from build123d import *

# Parameters (mm, degrees)
P_IDAT_VYSUNUT_M1_DEPTH  = 3
P_IDAT_VYSUNUT_M2_DEPTH  = 2
ZAOBLIT4_R               = 1
SKICA2_W                 = 4
SKICA2_H                 = 2
ODEBRAT_VYSUNUT_M2_DEPTH = 0.8
SKICA3_W                 = 4
SKICA3_H                 = 2
ODEBRAT_VYSUNUT_M3_DEPTH = 0.8


with BuildPart() as part:
    # Skica1 → P_idat vysunut_m1 (new body)
    with BuildSketch(Plane(origin=(0, 0, 0), x_dir=(1, 0, 0), z_dir=(0, 1, 0))):
        Polygon((-118.143750166, 15), (-118.143750166, 0), (-68.779346971, 32.313398106), (-16.32734533, 12.51119421), (-26.593132493, 30.830954414), (-20.343228113, 42.230019956), (0, 37.22), (0, 69.22), (-39.317553332, 46.52), (-78.635106664, 69.22), (-118.143185584, 46.41), (-118.143185584, 33.5570142), (-107.643750166, 37.378496169), (-107.643750166, 24.278496169), (-128.093750166, 24.278496169), (-128.093750166, 11.378496169), align=None)
    extrude(amount=P_IDAT_VYSUNUT_M1_DEPTH)

    # Skica1_5 → P_idat vysunut_m2 (add)
    with BuildSketch(Plane(origin=(0, 0, 0), x_dir=(1, 0, 0), z_dir=(0, 1, 0))):
        Polygon((-68.779346971, 32.313398106), (-118.143750166, 0), (0, 0), (0, 15), (9.950504516, 11.37831254), (9.950504516, 24.27831254), (-10.5, 24.27831254), (-10.5, 37.37831254), (0, 33.55662508), (0, 37.22), (-20.343228113, 42.230019956), (-26.593132493, 30.830954414), (-16.32734533, 12.51119421), align=None)
    extrude(amount=P_IDAT_VYSUNUT_M2_DEPTH)

    # Zaoblit4
    zaoblit4_edges = [part.edges().sort_by_distance(p)[0] for p in [
        (-118.143750166, 1.5, -15),
        (-128.093750166, 1.5, -11.378496169),
        (-128.093750166, 1.5, -24.278496169),
        (-107.643750166, 1.5, -24.278496169),
        (-107.643750166, 1.5, -37.378496169),
        (-118.143185584, 1.5, -33.5570142),
        (-10.5, 1, -24.27831254),
        (-10.5, 1, -37.37831254),
        (0, 1, -33.55662508),
        (0, 1, -15),
        (9.950504516, 1, -11.37831254),
        (9.950504516, 1, -24.27831254),
    ]]
    fillet(zaoblit4_edges, radius=ZAOBLIT4_R)

    # Skica2 → Odebrat vysunut_m2 (cut)
    with BuildSketch(Plane(origin=(0, 3, 0), x_dir=(1, 0, 0), z_dir=(0, 1, 0))):
        with Locations((-105.643750166, 32.914422166)):
            Rectangle(SKICA2_W, SKICA2_H)
        with Locations((-126.093750166, 20.342570172)):
            Rectangle(SKICA2_W, SKICA2_H)
        with Locations((-105.643750166, 28.314422166)):
            Rectangle(SKICA2_W, SKICA2_H)
    extrude(amount=-ODEBRAT_VYSUNUT_M2_DEPTH, mode=Mode.SUBTRACT)

    # Skica3 → Odebrat vysunut_m3 (cut)
    with BuildSketch(Plane(origin=(0, 2, 0), x_dir=(1, 0, 0), z_dir=(0, 1, 0))):
        with Locations((7.950504516, 15.742386544)):
            Rectangle(SKICA3_W, SKICA3_H)
    extrude(amount=-ODEBRAT_VYSUNUT_M3_DEPTH, mode=Mode.SUBTRACT)


solid = part.part
Part model, mm, in its own coordinate system. A direction names the side the tool comes from. Coordinates: 2 decimals unless noted, no trailing zeros. Loops run counter-clockwise (first coordinate to the right, second up) from the corner with the lowest first, then second, coordinate; pieces in that order, holes last. Notation, with made-up numbers: (74.25, -39.5) -> (132.25, -39.5) arc R3 ccw to (132.25, -34.5) -> close; hole circle Ø1 at (-19, 8.5). An arc over 180 degrees is marked (long way). Use a Markdown table: item, result. Add a question column.
Item 1: Which spindle directions (+Z, -Z, +X, -X, +Y, -Y) get a long thin tool onto all of the face, cutting with end or side? Do faces 1 (the flat face through (-5.305, 0.986, -35.487)), 2 (the flat face through (-123.17, 1.48, -13.17)), 3 (the flat face through (-93.81, 2.49, -15.93)). Say none if no direction does.
Item 2: Band-saw the part on C-C on x = -42.5. Write the cut outline in (y, z), plus the area to 3 significant figures.
Item 3: Pull direction X, two halves, no side cores. Call faces 4 (the flat face through (-60, 0, -27)), 5 (the flat face through (-107.644, 1, -31)), 6 (the flat face through (-21.388, 2.493, -21.543)), 7 (the flat face through (-118.143, 1, -41)): +X half, -X half, draft (parallel to the pull), parting line (faces both ways), or undercut.
Item 4: Flat gauge pins, fed straight in: P1, Ø0.9, axis at x = -106.5, y = 2.5, coming from the -Z side; P2, Ø0.6, axis at x = 1.5, y = 1, coming from the -Z side; P3, Ø1.5, axis at y = 1.5, z = -30, coming from the -X side. Where does each tip first touch, or does it go through?
Item 5: Band-saw the part on D-D on z = -5. Write the cut outline in (x, y), plus the area to 3 significant figures.
Item 6: Band-saw the part on B-B on z = -61.5. Write the cut outline in (x, y).
Item 7: Probe probe 1 along Y at (x, z) = (-39, -19); probe 2 along X at (y, z) = (2.45, -43); probe 3 along Z at (x, y) = (-114.5, 0.25). List the from-to ranges inside material, lowest first.
Geometry says:
| question | item | result |
|---|---|---|
| 1 | face 1 | +Y, -Y |
| 1 | face 2 | +Z, +Y, -Y |
| 1 | face 3 | +Z, +Y |
| 2 | outline | (0, -48.36) -> (3, -48.36) -> (3, -22.39) -> (2, -22.39) -> (2, 0) -> (0, 0) -> close |
| 2 | area | 123 mm² |
| 3 | face 4 | draft |
| 3 | face 5 | undercut |
| 3 | face 6 | +X half |
| 3 | face 7 | -X half |
| 4 | P1 | z = -53.39 |
| 4 | P2 | z = -24.28 |
| 4 | P3 | x = -107.64 |
| 5 | outline | (-118.14, 0) -> (0, 0) -> (0, 2) -> (-110.51, 2) -> (-110.51, 3) -> (-118.14, 3) -> close |
| 5 | area | 244 mm² |
| 6 | outline | (-92.01, 0) -> (-65.26, 0) -> (-65.26, 3) -> (-92.01, 3) -> close; (-13.37, 0) -> (0, 0) -> (0, 3) -> (-13.37, 3) -> close |
| 7 | probe 1 | 0 to 2 |
| 7 | probe 2 | -118.14 to 0 |
| 7 | probe 3 | -48.51 to -34.88, -24.28 to 0 |
